Could you check a few things on this model? Use its own coordinates, in mm. A direction names the side the tool comes from. Give positions to 0.01 mm unless a question says otherwise; leave off trailing zeros. Loops run counter-clockwise (first coordinate to the right, second up) from the corner with the lowest first, then second, coordinate; pieces in that order, holes last. Notation, with made-up numbers: (-14.75, 57) - (-3.75, 57) arc R30 ccw to (-3.75, 88) - close; hole circle Ø9 at (-24.5, -38). An arc over 180 degrees is marked (long way). Use CSV: the item, a comma, the result in double quotes.
from build123d import *

# Parameters (mm, degrees)
SKETCH1_W                = 228.6
SKETCH1_H                = 127
BOSS_EXTRUDE1_DEPTH      = 50.8
CUT_EXTRUDE24_DEPTH      = 196.514014843
CUT_EXTRUDE24_DEPTH_BACK = 196.514014843
SKETCH30_W               = 94.400264643
SKETCH30_H               = 127
SKETCH30_W_2             = 58.559389051
SKETCH31_W               = 75.640346306
SKETCH31_H               = 101.6
CUT_EXTRUDE25_DEPTH      = 68.58
CUT_EXTRUDE26_DEPTH      = 73.726300143
CUT_EXTRUDE26_DEPTH_BACK = 73.726300143
SKETCH32_OUTSIDE_W       = 113.175
SKETCH32_OUTSIDE_H       = 130.144
SKETCH32_OUTSIDE_R       = 50.8
SKETCH34_W               = 90.599470714
SKETCH34_H               = 139.7
SKETCH34_R               = 3.429
BOSS_EXTRUDE2_DEPTH      = 3.175
CUT_EXTRUDE28_DEPTH      = 91.882042278
CUT_EXTRUDE28_DEPTH_BACK = 91.882042278


with BuildPart() as part:
    # Sketch1 → Boss-Extrude1 (new, symmetric)
    with BuildSketch(Plane.XY):
        with Locations((-25.4, -63.5)):
            Rectangle(SKETCH1_W, SKETCH1_H)
    extrude(amount=BOSS_EXTRUDE1_DEPTH, both=True)

    # Sketch2 → Cut-Revolve1 (revolve, cut)
    with BuildSketch(Plane.XY, mode=Mode.PRIVATE) as cut_revolve1_sk:
        Polygon((-50.503182361, -16.903094944), (-105.996730082, 3.29490462), (-55.183426739, 142.903308162), (40.289343532, 108.1540616), (0, -2.54), (-14.86761563, -43.388438226), (-54.846838182, -28.837191228), align=None)
    revolve(cut_revolve1_sk.sketch.rotate(Axis((-60.4239625, -168.553472561, 0), (0.3420201433256656, 0.9396926207859095, 0)), 180), axis=Axis((-60.4239625, -168.553472561, 0), (0.3420201433256656, 0.9396926207859095, 0)), mode=Mode.SUBTRACT)

    # Sketch30 → Cut-Extrude24 (cut, two sides: drawn at the far end of the back side and taken through both)
    with BuildSketch(Plane.XY.offset(-CUT_EXTRUDE24_DEPTH_BACK)):
        with Locations((-92.499867679, -63.5)):
            Rectangle(SKETCH30_W, SKETCH30_H)
        with Locations((59.620305475, -63.5)):
            Rectangle(SKETCH30_W_2, SKETCH30_H)
    extrude(amount=CUT_EXTRUDE24_DEPTH + CUT_EXTRUDE24_DEPTH_BACK, mode=Mode.SUBTRACT)

    # Sketch31 → Cut-Extrude25 (cut)
    with BuildSketch(Plane.XZ.offset(127)):
        with Locations((-7.479562204, 0)):
            Rectangle(SKETCH31_W, SKETCH31_H)
    extrude(amount=-CUT_EXTRUDE25_DEPTH, mode=Mode.SUBTRACT)

    # Sketch32 outside → Cut-Extrude26 (cut, two sides: drawn at the far end of the back side and taken through both)
    with BuildSketch(Plane(origin=(-15.683955895, -43.091314668, 0), x_dir=(0.9396926207859096, -0.3420201433256657, 0), z_dir=(0.3420201433256657, 0.9396926207859096, 0)).offset(-CUT_EXTRUDE26_DEPTH_BACK)):
        with Locations((6.1765, 0)):
            Rectangle(SKETCH32_OUTSIDE_W, SKETCH32_OUTSIDE_H)
        with Locations((0.868731164, 2.54)):
            Circle(SKETCH32_OUTSIDE_R, mode=Mode.SUBTRACT)
    extrude(amount=CUT_EXTRUDE26_DEPTH + CUT_EXTRUDE26_DEPTH_BACK, mode=Mode.SUBTRACT)

    # Sketch34 → Boss-Extrude2 (add)
    with BuildSketch(Plane.XZ.offset(58.42)):
        Rectangle(SKETCH34_W, SKETCH34_H)
        with Locations(Location((-38.949735357, 63.5, 0), (0, 0, 270))):
            Circle(SKETCH34_R, mode=Mode.SUBTRACT)
        with Locations(Location((-26.249735357, 63.5, 0), (0, 0, 270))):
            Circle(SKETCH34_R, mode=Mode.SUBTRACT)
        with Locations(Location((-13.549735357, 63.5, 0), (0, 0, 270))):
            Circle(SKETCH34_R, mode=Mode.SUBTRACT)
        with Locations(Location((-0.849735357, 63.5, 0), (0, 0, 270))):
            Circle(SKETCH34_R, mode=Mode.SUBTRACT)
        with Locations(Location((11.850264643, 63.5, 0), (0, 0, 270))):
            Circle(SKETCH34_R, mode=Mode.SUBTRACT)
        with Locations(Location((24.550264643, 63.5, 0), (0, 0, 270))):
            Circle(SKETCH34_R, mode=Mode.SUBTRACT)
        with Locations(Location((-26.249735357, -63.5, 0), (0, 0, 270))):
            Circle(SKETCH34_R, mode=Mode.SUBTRACT)
        with Locations(Location((-13.549735357, -63.5, 0), (0, 0, 270))):
            Circle(SKETCH34_R, mode=Mode.SUBTRACT)
        with Locations(Location((-0.849735357, -63.5, 0), (0, 0, 270))):
            Circle(SKETCH34_R, mode=Mode.SUBTRACT)
        with Locations(Location((11.850264643, -63.5, 0), (0, 0, 270))):
            Circle(SKETCH34_R, mode=Mode.SUBTRACT)
        with Locations(Location((24.550264643, -63.5, 0), (0, 0, 270))):
            Circle(SKETCH34_R, mode=Mode.SUBTRACT)
        with Locations(Location((-38.949735357, -63.5, 0), (0, 0, 270))):
            Circle(SKETCH34_R, mode=Mode.SUBTRACT)
        Polygon((8.18326415, 23.631227188), (17.570519416, 30.368097404), (24.550264643, 23.631227188), (27.611749682, 8.577894095), (26.081007163, -20.911612947), (15.410103284, -35.988916053), (9.99990449, -28.4502645), align=None, mode=Mode.SUBTRACT)
    extrude(amount=-BOSS_EXTRUDE2_DEPTH)

    # Sketch35 → Cut-Extrude28 (cut, two sides: drawn at the far end of the back side and taken through both)
    with BuildSketch(Plane(origin=(0, -55.245, 0), x_dir=(1, 0, 0), z_dir=(0, 1, 0)).offset(-CUT_EXTRUDE28_DEPTH_BACK)):
        Polygon((30.340610949, 28.79845063), (30.340610949, 69.85), (45.299735357, 69.85), (45.299735357, -69.85), (30.340610949, -69.85), align=None)
    extrude(amount=CUT_EXTRUDE28_DEPTH + CUT_EXTRUDE28_DEPTH_BACK, mode=Mode.SUBTRACT)


solid = part.part
1) Suppose I cut it at B-B (z = -16.5). Please give me the cut outline in (x, y).
Answer below:
outline,"(-45.3, -58.42) - (30.34, -58.42) - (30.34, -46.33) - (26.33, -44.87) - (21.98, -56.8) - (-45.3, -32.31) - close"
2) Which directions (+Z, -Z, +X, -X, +Y, -Y) give clear straight access to the entire face, cutting with the end or side of a thin tool? Please do faces 4 (the cylindrical face through (15.733, -49.245, -42.97)), 5 (the cylindrical face through (1.5, -56.9, -61)), 6 (the flat face through (-16, -44, -50.8)).
Answer below:
face 4,"-Z, +X"
face 5,"+Y, -Y"
face 6,"-Z, +X, -X, +Y"
3) Suppose I cut it at C-C (x = 0.5). State how many separate pieces and enclosed holes the cut face has, plus the area to 3 significant figures.
Answer below:
separate pieces,"3"
enclosed holes,"0"
area,"1,230 mm2"
4) Suppose I cut it at A-A (z = -63.5). Please give me the cut outline in (x, y) (3 decimals), plus the area to 3 significant figures.
Answer below:
outline,"(-45.3, -58.42) - (-42.379, -58.42) - (-42.379, -55.245) - (-45.3, -55.245) - close; (-35.521, -58.42) - (-29.679, -58.42) - (-29.679, -55.245) - (-35.521, -55.245) - close; (-22.821, -58.42) - (-16.979, -58.42) - (-16.979, -55.245) - (-22.821, -55.245) - close; (-10.121, -58.42) - (-4.279, -58.42) - (-4.279, -55.245) - (-10.121, -55.245) - close; (2.579, -58.42) - (8.421, -58.42) - (8.421, -55.245) - (2.579, -55.245) - close; (15.279, -58.42) - (21.121, -58.42) - (21.121, -55.245) - (15.279, -55.245) - close; (27.979, -58.42) - (30.341, -58.42) - (30.341, -55.245) - (27.979, -55.245) - close"
area,"110 mm2"
5) I'm going to push flat-ended pins straight in: P1, Ø12, axis at x = -6, y = -31, coming from the +Z side; P2, Ø8, axis at x = -0.85, z = 63.5, coming from the +Y side (3 decimals); P3, Ø2, axis at x = 0, z = 30.5, coming from the +Y side. Where does each tip first touch, or does it pass through?
Answer below:
P1,"stops at z = 48.26"
P2,"stops at y = -55.245"
P3,"stops at y = -48.44"
6) We'd pull the mould along Y, two halves only. Please class faces 1 (the cylindrical face through (-11.2, -56.9, -61)), 2 (the cylindrical face through (-18.13, -43.12, 48.16)), 3 (the flat face through (-8, -58.42, 1)): +Y half, -Y half, draft (parallel to the pull), parting line (faces both ways), or undercut.
Answer below:
face 1,"draft"
face 2,"undercut"
face 3,"-Y half"
7) I need wall thicknesses on line 1 along Z through (x, y) = (26.5, -56); line 2 along Z through (x, y) = (-15, -33); line 3 along Z through (x, y) = (-42, -29.5). Which ranges of each line are inside material? Lowest first, please.
Answer below:
line 1,"z = -69.85 to -66.32, -60.68 to 60.68, 66.32 to 69.85"
line 2,"z = -50.8 to -42.39, 42.39 to 48.13"
line 3,"z = -43.35 to -29.92, 29.92 to 38.27"
